Check sheet for the modelled part. Datum: model origin and axes. Units: mm. Round coordinates to 2 decimals unless told otherwise and drop trailing zeros. Order: outer loops, then holes, each group sorted by start corner. A loop starts at its lowest first (then second) coordinate and runs counter-clockwise, first axis right, second up.
(1) Sectioned sample at C-C, the plane y = 1.3. Enter the section's corners in (x, z), and give its area (3 significant figures).
(2) Sectioned sample at B-B, the plane x = -17. Enter the section's corners in (y, z), and give its area (4 significant figures).
(3) Sectioned sample at A-A, the plane z = -40. Enter the section's corners in (x, y).
(4) Thickness scan on probe 1 along X at (y, z) = (3.7, -40); probe 2 along X at (y, z) = (3.9, 0); probe 3 along X at (y, z) = (1.6, 16). Record the ranges inside material, lowest first.
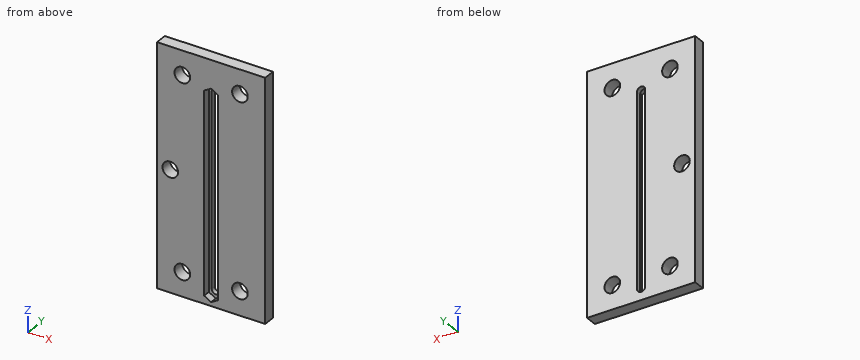
```python
from build123d import *

# Parameters (mm, degrees)
SKETCH1_W           = 45
SKETCH1_H           = 100
SKETCH1_R           = 3.25
BOSS_EXTRUDE1_DEPTH = 5
CUT_EXTRUDE1_DEPTH  = 2
CUT_EXTRUDE2_REACH  = 56.911


with BuildPart() as part:
    # Sketch1 → Boss-Extrude1 (new body)
    with BuildSketch(Plane(origin=(0, 0, 0), x_dir=(1, 0, 0), z_dir=(0, 1, 0))):
        Rectangle(SKETCH1_W, SKETCH1_H)
        with Locations(Location((-12, 40, 0), (0, 0, 270))):
            Circle(SKETCH1_R, mode=Mode.SUBTRACT)
        with Locations(Location((12, 40, 0), (0, 0, 270))):
            Circle(SKETCH1_R, mode=Mode.SUBTRACT)
        with Locations(Location((12, -40, 0), (0, 0, 270))):
            Circle(SKETCH1_R, mode=Mode.SUBTRACT)
        with Locations(Location((-12, -40, 0), (0, 0, 270))):
            Circle(SKETCH1_R, mode=Mode.SUBTRACT)
        with Locations(Location((-17, 0, 0), (0, 0, 270))):
            Circle(SKETCH1_R, mode=Mode.SUBTRACT)
    extrude(amount=BOSS_EXTRUDE1_DEPTH)

    # Sketch2 → Cut-Extrude1 (cut)
    with BuildSketch(Plane(origin=(0, 5, 0), x_dir=(1, 0, 0), z_dir=(0, 1, 0))):
        with BuildLine():
            Line((1.7, 45), (1.7, -35))
            ThreePointArc((1.7, -35), (0, -36.7), (-1.7, -35))
            Line((-1.7, -35), (-1.7, 45))
            ThreePointArc((-1.7, 45), (0, 46.7), (1.7, 45))
        make_face()
    extrude(amount=-CUT_EXTRUDE1_DEPTH, mode=Mode.SUBTRACT)

    # Sketch3 → Cut-Extrude2 (cut, up to next)
    with BuildSketch(Plane(origin=(0, 3, 0), x_dir=(1, 0, 0), z_dir=(0, 1, 0)), mode=Mode.PRIVATE) as cut_extrude2_sk1:
        with BuildLine():
            Line((0, 41.651368439), (1.7, 42.632863896))
            Line((1.7, 42.632863896), (1.7, 45))
            ThreePointArc((1.7, 45), (0, 46.7), (-1.7, 45))
            Line((-1.7, 45), (-1.7, 42.632863896))
            Line((-1.7, 42.632863896), (0, 41.651368439))
        make_face()
    cut_extrude2_tool1 = extrude(cut_extrude2_sk1.sketch, amount=-CUT_EXTRUDE2_REACH, mode=Mode.PRIVATE) & part.part
    # Sketch3 → Cut-Extrude2 (cut, up to next)
    with BuildSketch(Plane(origin=(0, 3, 0), x_dir=(1, 0, 0), z_dir=(0, 1, 0)), mode=Mode.PRIVATE) as cut_extrude2_sk2:
        Polygon((1.7, -32.632863896), (1.7, 42.632863896), (0, 41.651368439), (-1.7, 42.632863896), (-1.7, -32.632863896), (0, -31.651368439), align=None)
    cut_extrude2_tool2 = extrude(cut_extrude2_sk2.sketch, amount=-CUT_EXTRUDE2_REACH, mode=Mode.PRIVATE) & part.part
    # Sketch3 → Cut-Extrude2 (cut, up to next)
    with BuildSketch(Plane(origin=(0, 3, 0), x_dir=(1, 0, 0), z_dir=(0, 1, 0)), mode=Mode.PRIVATE) as cut_extrude2_sk3:
        with BuildLine():
            Line((1.7, -35), (1.7, -32.632863896))
            Line((1.7, -32.632863896), (0, -31.651368439))
            Line((0, -31.651368439), (-1.7, -32.632863896))
            Line((-1.7, -32.632863896), (-1.7, -35))
            ThreePointArc((-1.7, -35), (0, -36.7), (1.7, -35))
        make_face()
    cut_extrude2_tool3 = extrude(cut_extrude2_sk3.sketch, amount=-CUT_EXTRUDE2_REACH, mode=Mode.PRIVATE) & part.part
    # Sketch3 → Cut-Extrude2 (cut, up to next)
    with BuildSketch(Plane(origin=(0, 3, 0), x_dir=(1, 0, 0), z_dir=(0, 1, 0)), mode=Mode.PRIVATE) as cut_extrude2_sk4:
        Polygon((-1.7, -32.632863896), (-1.7, 42.632863896), (-2.9, 43.325684219), (-2.9, -33.325684219), align=None)
    cut_extrude2_tool4 = extrude(cut_extrude2_sk4.sketch, amount=-CUT_EXTRUDE2_REACH, mode=Mode.PRIVATE) & part.part
    # Sketch3 → Cut-Extrude2 (cut, up to next)
    with BuildSketch(Plane(origin=(0, 3, 0), x_dir=(1, 0, 0), z_dir=(0, 1, 0)), mode=Mode.PRIVATE) as cut_extrude2_sk5:
        Polygon((2.9, -33.325684219), (2.9, 43.325684219), (1.7, 42.632863896), (1.7, -32.632863896), align=None)
    cut_extrude2_tool5 = extrude(cut_extrude2_sk5.sketch, amount=-CUT_EXTRUDE2_REACH, mode=Mode.PRIVATE) & part.part
    # Sketch3 → Cut-Extrude2 (cut, up to next)
    with BuildSketch(Plane(origin=(0, 3, 0), x_dir=(1, 0, 0), z_dir=(0, 1, 0)), mode=Mode.PRIVATE) as cut_extrude2_sk6:
        with BuildLine():
            Line((1.7, 42.632863896), (2.9, 43.325684219))
            Line((2.9, 43.325684219), (2.9, 46.674315781))
            Line((2.9, 46.674315781), (0, 48.348631561))
            Line((0, 48.348631561), (-2.9, 46.674315781))
            Line((-2.9, 46.674315781), (-2.9, 43.325684219))
            Line((-2.9, 43.325684219), (-1.7, 42.632863896))
            Line((-1.7, 42.632863896), (-1.7, 45))
            ThreePointArc((-1.7, 45), (0, 46.7), (1.7, 45))
            Line((1.7, 45), (1.7, 42.632863896))
        make_face()
    cut_extrude2_tool6 = extrude(cut_extrude2_sk6.sketch, amount=-CUT_EXTRUDE2_REACH, mode=Mode.PRIVATE) & part.part
    # Sketch3 → Cut-Extrude2 (cut, up to next)
    with BuildSketch(Plane(origin=(0, 3, 0), x_dir=(1, 0, 0), z_dir=(0, 1, 0)), mode=Mode.PRIVATE) as cut_extrude2_sk7:
        with BuildLine():
            Line((2.9, -36.674315781), (2.9, -33.325684219))
            Line((2.9, -33.325684219), (1.7, -32.632863896))
            Line((1.7, -32.632863896), (1.7, -35))
            ThreePointArc((1.7, -35), (0, -36.7), (-1.7, -35))
            Line((-1.7, -35), (-1.7, -32.632863896))
            Line((-1.7, -32.632863896), (-2.9, -33.325684219))
            Line((-2.9, -33.325684219), (-2.9, -36.674315781))
            Line((-2.9, -36.674315781), (0, -38.348631561))
            Line((0, -38.348631561), (2.9, -36.674315781))
        make_face()
    cut_extrude2_tool7 = extrude(cut_extrude2_sk7.sketch, amount=-CUT_EXTRUDE2_REACH, mode=Mode.PRIVATE) & part.part
    add(cut_extrude2_tool1.solids().sort_by_distance((0, 3, -44.246241))[0], mode=Mode.SUBTRACT)
    add(cut_extrude2_tool2.solids().sort_by_distance((0, 3, -5))[0], mode=Mode.SUBTRACT)
    add(cut_extrude2_tool3.solids().sort_by_distance((0, 3, 34.246241))[0], mode=Mode.SUBTRACT)
    add(cut_extrude2_tool4.solids().sort_by_distance((-2.301824, 3, -5))[0], mode=Mode.SUBTRACT)
    add(cut_extrude2_tool5.solids().sort_by_distance((2.301824, 3, -5))[0], mode=Mode.SUBTRACT)
    add(cut_extrude2_tool6.solids().sort_by_distance((2.259285, 3, -43.049795))[0], mode=Mode.SUBTRACT)
    add(cut_extrude2_tool7.solids().sort_by_distance((1.409285, 3, 37.440952))[0], mode=Mode.SUBTRACT)


solid = part.part
```
Derived:
1. outline: (-22.5, -50) - (22.5, -50) - (22.5, 50) - (-22.5, 50) - close; hole circle Ø6.5 at (-17, 0); hole circle Ø6.5 at (-12, -40); hole circle Ø6.5 at (-12, 40); hole (-2.9, -46.67) - (0, -48.35) - (2.9, -46.67) - (2.9, 36.67) - (0, 38.35) - (-2.9, 36.67) - close; hole circle Ø6.5 at (12, -40); hole circle Ø6.5 at (12, 40)
1. area: 3,840 mm2
2. outline: (0, -50) - (5, -50) - (5, -3.25) - (0, -3.25) - close; (0, 3.25) - (5, 3.25) - (5, 50) - (0, 50) - close
2. area: 467.5 mm2
3. outline: (-22.5, 0) - (-15.25, 0) - (-15.25, 5) - (-22.5, 5) - close; (-8.75, 0) - (-2.9, 0) - (-2.9, 3) - (-1.7, 3) - (-1.7, 5) - (-8.75, 5) - close; (1.7, 3) - (2.9, 3) - (2.9, 0) - (8.75, 0) - (8.75, 5) - (1.7, 5) - close; (15.25, 0) - (22.5, 0) - (22.5, 5) - (15.25, 5) - close
4. probe 1: x = -22.5 to -15.25, -8.75 to -1.7, 1.7 to 8.75, 15.25 to 22.5
4. probe 2: x = -22.5 to -20.25, -13.75 to -1.7, 1.7 to 22.5
4. probe 3: x = -22.5 to -2.9, 2.9 to 22.5
